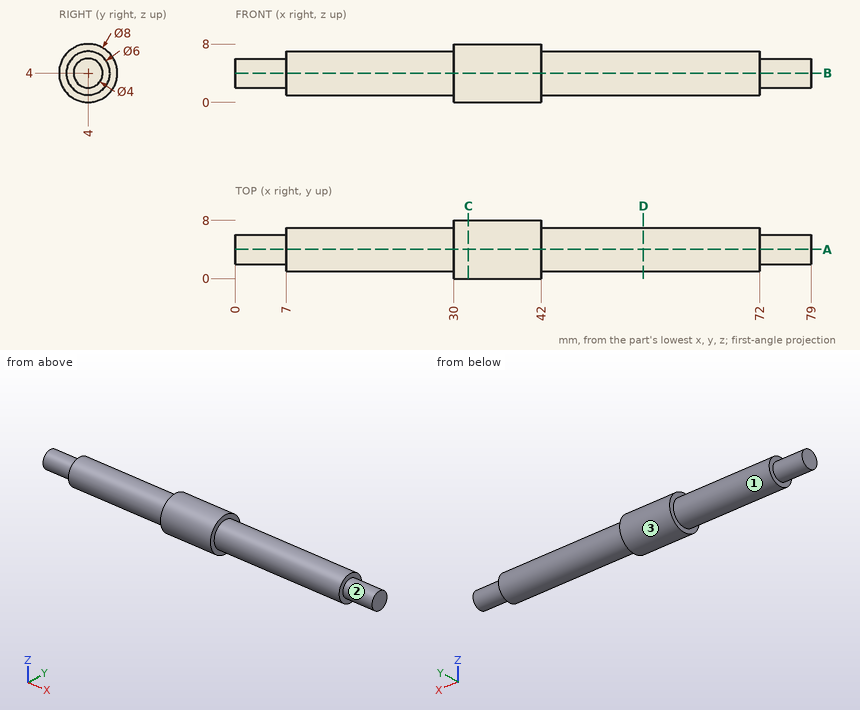
Geometry: see drawing. Coordinates: mm, zero at the bounding-box minimum. A direction names the side the tool comes from. Round coordinates to 2 decimals unless told otherwise and drop trailing zeros. Loops run counter-clockwise (first coordinate to the right, second up) from the corner with the lowest first, then second, coordinate; pieces in that order, holes last. Notation, with made-up numbers: M 37,68 L 69,68 A23 ccw 69,93 Z; hole C -38.5,15.25 d5. An arc over 180 degrees is marked long. Use a Markdown table: item, result. Add a question column.
1. Line query: line 1 (X direction, y = 2.25, z = 2.5); line 2 (X direction, y = 3, z = 7.75); line 3 (Z direction, x = 57, y = 4.25). Output: solid intervals per line, ascending.
2. Section query A-A on y = 4. Return the cut outline in (x, z).
3. Contact query for a flat-ended pin moving along its axis: P1, Ø1, axis at x = 62, y = 1, coming from the +Z side. Output: stop coordinate, or through.
4. Section query D-D on x = 56. Return the cut outline in (y, z).
5. Section query C-C on x = 32. Return the cut outline in (y, z), then the cut area to 3 significant figures.
6. Reachability of the marked faces 1, 2 and 3 from +Z, -Z, +X, -X, +Y, -Y: full face, straight path, thin tool, end or side. Return the list, or none.
Reported:
| question | item | result |
|---|---|---|
| 1 | line 1 | x = 7 to 72 |
| 1 | line 2 | x = 30 to 42 |
| 1 | line 3 | z = 1.01 to 6.99 |
| 2 | outline | M 0,2 L 7,2 L 7,1 L 30,1 L 30,0 L 42,0 L 42,1 L 72,1 L 72,2 L 79,2 L 79,6 L 72,6 L 72,7 L 42,7 L 42,8 L 30,8 L 30,7 L 7,7 L 7,6 L 0,6 Z |
| 3 | P1 | stops at z = 5.66 |
| 4 | outline | C 4,4 d6 |
| 5 | outline | C 4,4 d8 |
| 5 | area | 50.3 mm² |
| 6 | face 1 | -X |
| 6 | face 2 | +X |
| 6 | face 3 | +X, -X |
